from build123d import *

# Parameters (mm, degrees)
SKETCH1_R           = 5
BOSS_EXTRUDE1_DEPTH = 6
BOSS_EXTRUDE1_TAPER = 4
CUT_EXTRUDE1_DEPTH  = 4
SKETCH4_R           = 1.65
CUT_EXTRUDE2_DEPTH  = 9.124038405


with BuildPart() as part:
    # Sketch1 → Boss-Extrude1 (new body)
    with BuildSketch(Plane.XY):
        Circle(SKETCH1_R)
    extrude(amount=BOSS_EXTRUDE1_DEPTH, taper=BOSS_EXTRUDE1_TAPER)

    # Sketch2 → Cut-Extrude1 (cut)
    with BuildSketch(Plane.XY.offset(6)):
        Polygon((1.732050808, 3), (-1.732050808, 3), (-3.464101615, 0), (-1.732050808, -3), (1.732050808, -3), (3.464101615, 0), align=None)
    extrude(amount=-CUT_EXTRUDE1_DEPTH, mode=Mode.SUBTRACT)

    # Sketch4 → Cut-Extrude2 (cut, through all)
    with BuildSketch(Plane.XY.offset(2)):
        Circle(SKETCH4_R)
    extrude(amount=-CUT_EXTRUDE2_DEPTH, mode=Mode.SUBTRACT)


solid = part.part
Geometry check sheet. Reference: the model listing, model coordinates, mm. A direction names the side the tool comes from. Give positions to 0.01 mm unless a question says otherwise; leave off trailing zeros. Loops run counter-clockwise (first coordinate to the right, second up) from the corner with the lowest first, then second, coordinate; pieces in that order, holes last. Notation, with made-up numbers: M 30.5,42 L 56.5,42 A17 cw 56.5,54 Z; hole C 20,89.25 d10. An arc over 180 degrees is marked long. Answer as a JSON object with one key per item and string values. Group by question number.
Item 1: Sectioned sample at A-A on x = 0. Record the boundary of the cut face in (y, z), plus the area to 3 significant figures.
Item 2: Mould release check, pull along Y, two halves, no side actions. Record for faces 1 (the conical face through (-0.623, 4.747, 3.042)), 2 (the cylindrical face through (-1.216, 1.115, 1.014)), 3 (the flat face through (2, 0, 0)): pulls with the +Y half, pulls with the -Y half, needs draft (parallel to the pull), parting line crosses it, or undercut.
Item 3: Sectioned sample at C-C on z = 1. Record the boundary of the cut face in (x, y).
Item 4: Sectioned sample at D-D on z = 1.75. Record the boundary of the cut face in (x, y).
Item 5: Access from +Z, -Z, +X, -X, +Y, -Y to the whole of each face (thin tool, end or side, straight path). Record for faces 4 (the flat face through (-2.6, -1.5, 4)), 5 (the flat face through (-3.1, 1.1, 6)).
Item 6: Gauge pin test, flat ends, axial feed: pin 1 (1 mm diameter, centred on x = 2.5, z = 2.5, fed in from +Y); pin 2 (3 mm diameter, centred on x = 2, y = -1, fed in from -Z); pin 3 (3 mm diameter, centred on x = -0.5, y = 0, fed in from +Z); pin 4 (1.7 mm diameter, centred on x = 0.5, z = 3.5, fed in from +Y). Record the tip position at first contact, or that the pin passes through.
Item 7: Sectioned sample at B-B on z = 2.75. Record the boundary of the cut face in (x, y), plus the area to 3 significant figures.
Item 8: Material ranges on L1, parallel to Z at x = -0.5, y = -2.75; L2, parallel to Y at x = -1.5, z = 5.25; L3, parallel to Y at x = -0.75, z = 3.5, recorded low to high.
Findings below:
{
 "1": {"outline": "M -5,0 L -1.65,0 L -1.65,2 L -3,2 L -3,6 L -4.58,6 Z; M 1.65,0 L 5,0 L 4.58,6 L 3,6 L 3,2 L 1.65,2 Z", "area": "26.9 mm2"},
 "2": {"face 1": "parting line crosses it", "face 2": "undercut", "face 3": "needs draft"},
 "3": {"outline": "C 0,0 d9.86; hole C 0,0 d3.3"},
 "4": {"outline": "C 0,0 d9.76; hole C 0,0 d3.3"},
 "5": {"face 4": "+Z", "face 5": "+Z, +X, -X, +Y, -Y"},
 "6": {"pin 1": "y = 4.39", "pin 2": "z = 0", "pin 3": "z = 2", "pin 4": "y = 4.81"},
 "7": {"outline": "C 0,0 d9.62; hole M -3.46,0 L -1.73,-3 L 1.73,-3 L 3.46,0 L 1.73,3 L -1.73,3 Z", "area": "41.4 mm2"},
 "8": {"L1": "0 to 2", "L2": "-4.38 to -3, 3 to 4.38", "L3": "-4.7 to -3, 3 to 4.7"}
}
